Design review of the part built by this model. Coordinates are the model's own, in mm. A direction names the side the tool comes from. Coordinates: 2 decimals unless noted, no trailing zeros. Write each loop counter-clockwise with the first axis right and the second up, starting at its lowest first coordinate (ties: lowest second). Pieces come first, ordered by that corner, then holes. Notation, with made-up numbers: (-40, -8) -> (-33, -8) arc R20 cw to (-33, 31) -> close; hole circle Ø5 at (26.25, 26). An arc over 180 degrees is marked (long way). One line per question, with ' | ' between items. Start each with the question number.
Q1. Add section D-D on y = 457.2. State the section outline as (x, z) points (3 decimals), and give its area (3 significant figures).
Q2. For P1, Ø11.5, axis at x = -24.5, z = 212.5, coming from the +Y side; P2, Ø21.5, axis at y = 457.2, z = 76.2, coming from the +X side; P3, Ø10, axis at y = 398.5, z = 174.5, coming from the -X side (3 decimals); P4, Ø5.5, axis at x = 1.5, y = 447, coming from the +Z side, all flat-tipped, find the tip position at first contact; note any pin that passes through.
Q3. Add section A-A on x = -81.5. State the section outline as (y, z) points.
Q4. Add section B-B on y = -119. State the section outline as (x, z) points (3 decimals).
Q5. Add section C-C on z = 76.2. State the section outline as (x, y) points (3 decimals), and give its area (3 significant figures).
Q6. Wall thickness on probe 1 along Z at (x, y) = (-2, 457.2); probe 2 along Z at (x, y) = (47, -404); probe 3 along X at (y, z) = (103.5, 133) (3 decimals): over which ranges is each line inside the solid? List them lowest first.
Q7. For faces 5 (the flat face through (-1, -508, 35)), 6 (the flat face through (0, 433, 190.5)), 7 (the flat face through (-69, -7, -203.2)), 8 (the flat face through (69, -82, 203.2)), 9 (the cylindrical face through (-0.13, 470.68, 0.59)), list the 3-axis set-ups (+Z, -Z, +X, -X, +Y, -Y) from which the entire face can be reached by the end or side of a thin tool; tool diameter is ignored.
Q8. Draft analysis for pull direction Y (two halves, no side actions). For faces 1 (the flat face through (-127, -7, -216)), 2 (the cylindrical face through (-0.13, 470.68, 152.99)), 3 (the flat face through (-1, 508, -111)), 4 (the cylindrical face through (-0.133, 467.145, -67.08)), state which applies: pulls with the +Y half, pulls with the -Y half, needs draft (parallel to the pull), parting line crosses it, or undercut.
from build123d import *

# Parameters (mm, degrees)
F1_DEPTH = 508
F3_D     = 26.9875
F4_W     = 254
F4_H     = 152.4
F5_DEPTH = 38.1


with BuildPart() as f1:
    # F0 (on Front) → F1 (new body, symmetric)
    with BuildSketch(Plane.XZ):
        with BuildLine():
            Line((127, -228.6), (127, -203.2))
            Line((127, -203.2), (12.065, -203.2))
            ThreePointArc((12.065, -203.2), (10.268949, -202.456051), (9.525, -200.66))
            Line((9.525, -200.66), (9.525, 200.66))
            ThreePointArc((9.525, 200.66), (10.268949, 202.456051), (12.065, 203.2))
            Line((12.065, 203.2), (127, 203.2))
            Line((127, 203.2), (127, 228.6))
            Line((127, 228.6), (-127, 228.6))
            Line((-127, 228.6), (-127, 203.2))
            Line((-127, 203.2), (-12.065, 203.2))
            ThreePointArc((-12.065, 203.2), (-10.268949, 202.456051), (-9.525, 200.66))
            Line((-9.525, 200.66), (-9.525, -200.66))
            ThreePointArc((-9.525, -200.66), (-10.268949, -202.456051), (-12.065, -203.2))
            Line((-12.065, -203.2), (-127, -203.2))
            Line((-127, -203.2), (-127, -228.6))
            Line((-127, -228.6), (127, -228.6))
        make_face()
    extrude(amount=F1_DEPTH, both=True)

    # F3 (through all)
    with Locations(Plane.YZ.offset(9.525)):
        with Locations((457.2, 152.4), (457.2, 76.2), (457.2, 0), (457.2, -76.2)):
            Hole(F3_D / 2)

    # F4 (on face) → F5 (cut)
    with BuildSketch(Plane.XY.offset(228.6)):
        with Locations((0, 431.8)):
            Rectangle(F4_W, F4_H)
    extrude(amount=-F5_DEPTH, mode=Mode.SUBTRACT)


solid = f1.part
Output values:
1) outline: (-127, -228.6) -> (127, -228.6) -> (127, -203.2) -> (12.065, -203.2) arc R2.54 cw to (9.525, -200.66) -> (9.525, -89.694) -> (-9.525, -89.694) -> (-9.525, -200.66) arc R2.54 cw to (-12.065, -203.2) -> (-127, -203.2) -> close; (-9.525, -62.706) -> (9.525, -62.706) -> (9.525, -13.494) -> (-9.525, -13.494) -> close; (-9.525, 13.494) -> (9.525, 13.494) -> (9.525, 62.706) -> (-9.525, 62.706) -> close; (-9.525, 89.694) -> (9.525, 89.694) -> (9.525, 138.906) -> (-9.525, 138.906) -> close; (-9.525, 165.894) -> (9.525, 165.894) -> (9.525, 190.5) -> (-9.525, 190.5) -> close | area: 11,900 mm2
2) P1: stops at y = 355.6 | P2: passes through | P3: stops at x = -9.525 | P4: stops at z = 190.5
3) outline: (-508, -228.6) -> (508, -228.6) -> (508, -203.2) -> (-508, -203.2) -> close; (-508, 203.2) -> (355.6, 203.2) -> (355.6, 228.6) -> (-508, 228.6) -> close
4) outline: (-127, -228.6) -> (127, -228.6) -> (127, -203.2) -> (12.065, -203.2) arc R2.54 cw to (9.525, -200.66) -> (9.525, 200.66) arc R2.54 cw to (12.065, 203.2) -> (127, 203.2) -> (127, 228.6) -> (-127, 228.6) -> (-127, 203.2) -> (-12.065, 203.2) arc R2.54 cw to (-9.525, 200.66) -> (-9.525, -200.66) arc R2.54 cw to (-12.065, -203.2) -> (-127, -203.2) -> close
5) outline: (-9.525, -508) -> (9.525, -508) -> (9.525, 443.706) -> (-9.525, 443.706) -> close; (-9.525, 470.694) -> (9.525, 470.694) -> (9.525, 508) -> (-9.525, 508) -> close | area: 18,800 mm2
6) probe 1: z = -228.6 to -89.69, -62.71 to -13.49, 13.49 to 62.71, 89.69 to 138.91, 165.89 to 190.5 | probe 2: z = -228.6 to -203.2, 203.2 to 228.6 | probe 3: x = -9.525 to 9.525
7) face 5: +Z, -Z, +X, -X, -Y | face 6: +Z, +X, -X, +Y | face 7: -X, +Y, -Y | face 8: +X, +Y, -Y | face 9: +X, -X
8) face 1: needs draft | face 2: undercut | face 3: pulls with the +Y half | face 4: undercut
